Can you work these out from the model? Positions are in its coordinate system, mm. Face numbers are marked on the shaded views. Give positions to 0.01 mm unless a question says otherwise; leave off trailing zeros. Loops run counter-clockwise (first coordinate to the right, second up) from the corner with the lowest first, then second, coordinate; pieces in that order, holes last. Notation, with made-up numbers: (41, 68) -> (53, 68) arc R16 ccw to (53, 96) -> close; hole circle Ø8 at (-30.75, -28.75). An arc over 180 degrees is marked (long way). Return JSON: item names as keys, results as strings. Group by question number.
Q1. Suppose I cut it at C-C, the plane y = 2.25. Please give me the cut outline in (x, z), and give its area (3 significant figures).
Q2. I need wall thicknesses on line 1 along Y through (x, z) = (0, 3.6) (3 decimals); line 2 along X through (y, z) = (-1.25, 4.5); line 3 along Y through (x, z) = (1.05, 3). Which ranges of each line are inside material? Lowest first, please. Write a range as [from, to].
Q3. Thinking about a two-plate mould opening in Y: for the marked faces 1, 2, 3 and 4, which applies, pulls with the +Y half, pulls with the -Y half, needs draft (parallel to the pull), parting line crosses it, or undercut?
Q4. Suppose I cut it at A-A, the plane z = 6.5. Please give me the cut outline in (x, y) (3 decimals), and give its area (3 significant figures).
Q5. Will these pins go through, and if not, where does the flat tip stop? pin 1 (2 mm diameter, centred on x = -1.5, y = 0, fed in from -Z); pin 2 (1.5 mm diameter, centred on x = 0.5, z = 2.5, fed in from -Y) (3 decimals); pin 3 (3 mm diameter, centred on x = 1.5, z = 5.5, fed in from +Y) (3 decimals); pin 4 (2.5 mm diameter, centred on x = 0, y = 0, fed in from +Z).
Q6. Suppose I cut it at B-B, the plane x = 2.4. Please give me the cut outline in (y, z).
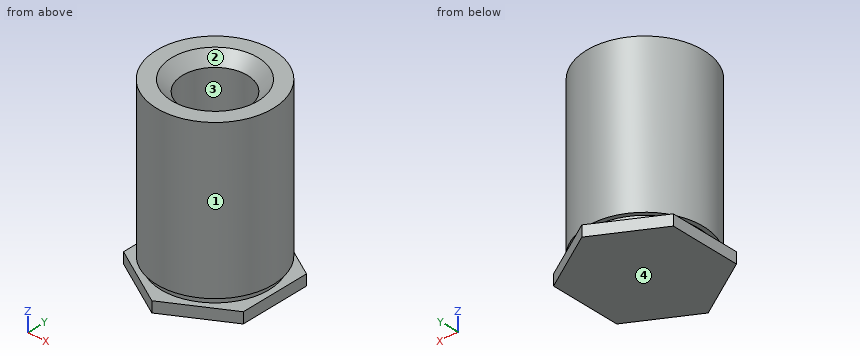
```python
from build123d import *

# Parameters (mm, degrees)
F1_DEPTH       = 0.5
F2_R           = 2.5
F3_DEPTH       = 0.3
F4_R           = 2.695
F5_DEPTH       = 7.2
F7_D           = 3
F7_DEPTH       = 5.4
F7_CSINK_D     = 4
F7_CSINK_ANGLE = 90
F7_TIP         = 0.9012909285


with BuildPart() as f1:
    # F0 (on Top) → F1 (new body)
    with BuildSketch(Plane.XY):
        Polygon((-2.7712812921, -1.6), (0, -3.2), (2.7712812921, -1.6), (2.7712812921, 1.6), (0, 3.2), (-2.7712812921, 1.6), align=None)
    extrude(amount=F1_DEPTH)

    # F2 (on face) → F3 (join)
    with BuildSketch(Plane.XY.offset(0.5)):
        Circle(F2_R)
    extrude(amount=F3_DEPTH)

    # F4 (on face) → F5 (join)
    with BuildSketch(Plane.XY.offset(0.8)):
        Circle(F4_R)
    extrude(amount=F5_DEPTH)

    # F7
    with Locations(Plane.XY.offset(8)):
        with Locations((0, 0)):
            CounterSinkHole(F7_D / 2, F7_CSINK_D / 2, depth=F7_DEPTH, counter_sink_angle=F7_CSINK_ANGLE)
            with Locations((0, 0, -(F7_DEPTH + F7_TIP / 2))):  # 118° drill point
                Cone(0, F7_D / 2, F7_TIP, mode=Mode.SUBTRACT)


solid = f1.part
```
Ans:
{
 "1": {"outline": "(-1.65, 0) -> (1.65, 0) -> (1.65, 0.5) -> (1.09, 0.5) -> (1.09, 0.8) -> (1.48, 0.8) -> (1.48, 8) -> (-1.48, 8) -> (-1.48, 0.8) -> (-1.09, 0.8) -> (-1.09, 0.5) -> (-1.65, 0.5) -> close", "area": "23.7 mm^2"},
 "2": {"line 1": "y = [-2.695, -1.5], [1.5, 2.695]", "line 2": "x = [-2.39, -0.83], [0.83, 2.39]", "line 3": "y = [-2.48, -1.07], [1.07, 2.48]"},
 "3": {"face 1": "parting line crosses it", "face 2": "undercut", "face 3": "undercut", "face 4": "needs draft"},
 "4": {"outline": "circle Ø5.39 at (0, 0); hole circle Ø3 at (0, 0)", "area": "15.7 mm^2"},
 "5": {"pin 1": "stops at z = 0", "pin 2": "stops at y = -2.695", "pin 3": "stops at y = 2.695", "pin 4": "stops at z = 2.45"},
 "6": {"outline": "(-1.81, 0) -> (1.81, 0) -> (1.81, 0.5) -> (0.7, 0.5) -> (0.7, 0.8) -> (1.23, 0.8) -> (1.23, 8) -> (-1.23, 8) -> (-1.23, 0.8) -> (-0.7, 0.8) -> (-0.7, 0.5) -> (-1.81, 0.5) -> close"}
}
